Autodesk Fusion 360 part; units mm, degrees
sketch "Sketch1" plane through (0, 0, 0) normal (0, 0, 1) x (1, 0, 0)
  line L0 (22.5, 4.5) -> (-22.5, 4.5)
  line L1 (-22.5, 4.5) -> (-22.5, -4.5)
  line L2 (-22.5, -4.5) -> (22.5, -4.5)
  line L3 (22.5, -4.5) -> (22.5, 4.5)
  line L4 (22.5, 4.5) -> (-22.5, -4.5) construction
  line L5 (-22.5, 4.5) -> (22.5, -4.5) construction
  dimension "d1" = 45
  dimension "d2" = 9
extrude "Extrude1" add sketch "Sketch1" along normal blind 2
fillet "Fillet1" radius 2.5 4 edges at (-22.5, -4.5, 1) (-22.5, 4.5, 1) (22.5, -4.5, 1) (22.5, 4.5, 1)
sketch "Sketch2" plane through (0, 0, 2) normal (0, 0, 1) x (-1, 0, 0)
  arc A0 (-22.5, -2) -> (-20, -4.5) centre (-20, -2) ccw
  line L0 (-20, -4.5) -> (20, -4.5)
  arc A1 (20, -4.5) -> (22.5, -2) centre (20, -2) ccw
  line L1 (20, 4.5) -> (-20, 4.5)
  line L2 (22.5, -2) -> (22.5, 2)
  arc A2 (22.5, 2) -> (20, 4.5) centre (20, 2) ccw
  arc A3 (-20, 4.5) -> (-22.5, 2) centre (-20, 2) ccw
  line L3 (-22.5, 2) -> (-22.5, -2)
  line L4 (22.5, 0) -> (-22.5, 0) construction
  line L5 (22.5, 0) -> (18, 0)
  line L6 (-22.5, 0) -> (-18, 0)
  circle A4 centre (18, 0) radius 2.7
  circle A5 centre (-18, 0) radius 2.7
  dimension "d11" = 4.5
  dimension "d12" = 4.5
  dimension "d13" = 5.4
  dimension "d14" = 5.4
extrude "Extrude2" cut sketch "Sketch2" against normal blind 2 contours A4 | A5
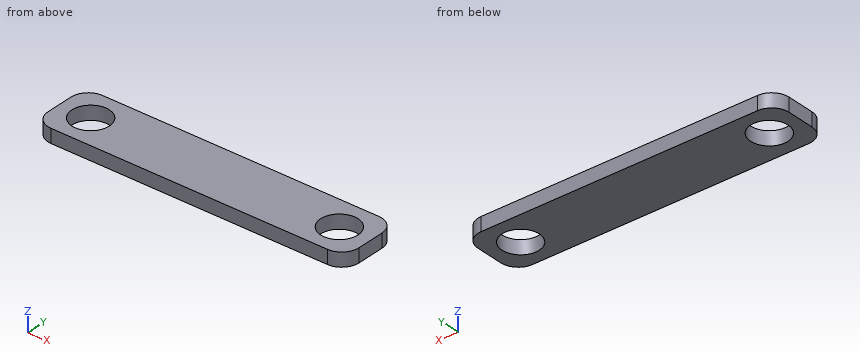
For this review, take the finished solid that the model builds, in its own axes (mm). Round coordinates to 2 decimals unless told otherwise and drop trailing zeros. Loops run counter-clockwise (first coordinate to the right, second up) from the corner with the lowest first, then second, coordinate; pieces in that order, holes last. Notation, with made-up numbers: (77.25, 29) - (128.25, 29) arc R24 cw to (128.25, 44) - close; hole circle Ø6 at (-27, 17). An arc over 180 degrees is marked (long way). Use one line per item in the form item = value.
1) Wall thickness on probe 1 along X at (y, z) = (0, 1.3); probe 2 along Y at (x, z) = (18, 1.2); probe 3 along X at (y, z) = (-1, 0.45): over which ranges is each line inside the solid? List them lowest first.
Solutions:
probe_1 = -22.5 to -20.7, -15.3 to 15.3, 20.7 to 22.5
probe_2 = -4.5 to -2.7, 2.7 to 4.5
probe_3 = -22.5 to -20.51, -15.49 to 15.49, 20.51 to 22.5
2) We need section B-B on y = 0. Write out the cut boundary in (x, z), then the cut area to 3 significant figures.
Solutions:
outline = (-22.5, 0) - (-20.7, 0) - (-20.7, 2) - (-22.5, 2) - close; (-15.3, 0) - (15.3, 0) - (15.3, 2) - (-15.3, 2) - close; (20.7, 0) - (22.5, 0) - (22.5, 2) - (20.7, 2) - close
area = 68.4 mm2
3) We need section C-C on z = 0.85. Write out the cut boundary in (x, y).
Solutions:
outline = (-22.5, -2) arc R2.5 ccw to (-20, -4.5) - (20, -4.5) arc R2.5 ccw to (22.5, -2) - (22.5, 2) arc R2.5 ccw to (20, 4.5) - (-20, 4.5) arc R2.5 ccw to (-22.5, 2) - close; hole circle Ø5.4 at (-18, 0); hole circle Ø5.4 at (18, 0)
4) We need section A-A on x = 18. Write out the cut boundary in (y, z), then the cut area to 3 significant figures.
Solutions:
outline = (-4.5, 0) - (-2.7, 0) - (-2.7, 2) - (-4.5, 2) - close; (2.7, 0) - (4.5, 0) - (4.5, 2) - (2.7, 2) - close
area = 7.20 mm2
5) We need section D-D on x = -16. Write out the cut boundary in (y, z).
Solutions:
outline = (-4.5, 0) - (-1.81, 0) - (-1.81, 2) - (-4.5, 2) - close; (1.81, 0) - (4.5, 0) - (4.5, 2) - (1.81, 2) - close
